Here's the drawing with two shaded views (mm, measured from the low corner). I have some questions. Round coordinates to 2 decimals unless told otherwise and drop trailing zeros. Loops run counter-clockwise (first coordinate to the right, second up) from the corner with the lowest first, then second, coordinate; pieces in that order, holes last.
(1) I want a section at A-A on y = 11.43. Write out the boundary of the cut face in (x, z), plus the area to 3 significant figures.
(2) I want a section at C-C on x = 4. Write out the boundary of the cut face in (y, z), plus the area to 3 significant figures.
(3) If I drill on line 1 along Z through (x, y) = (3.25, 11.43); line 2 along Y through (x, z) = (2.75, 17); line 3 along Y through (x, z) = (1.25, 10.75), over which ranges is the centre line in solid material (lowest first)?
(4) Thinking about a two-plate mould opening in Z: for the marked faces 1, 2 and 3, which applies, released by +Z, released by -Z, zero draft, split by the parting line, or undercut?
(5) Will these pins go through, and if not, where does the flat tip stop? pin 1 Ø1 at (x, y) = (3.5, 12.5) entering from -Z; pin 2 Ø1 at (x, y) = (3, 16.5) entering from +Z.
(6) I want a section at D-D on z = 20.5. Write out the boundary of the cut face in (x, y), plus the area to 3 significant figures.
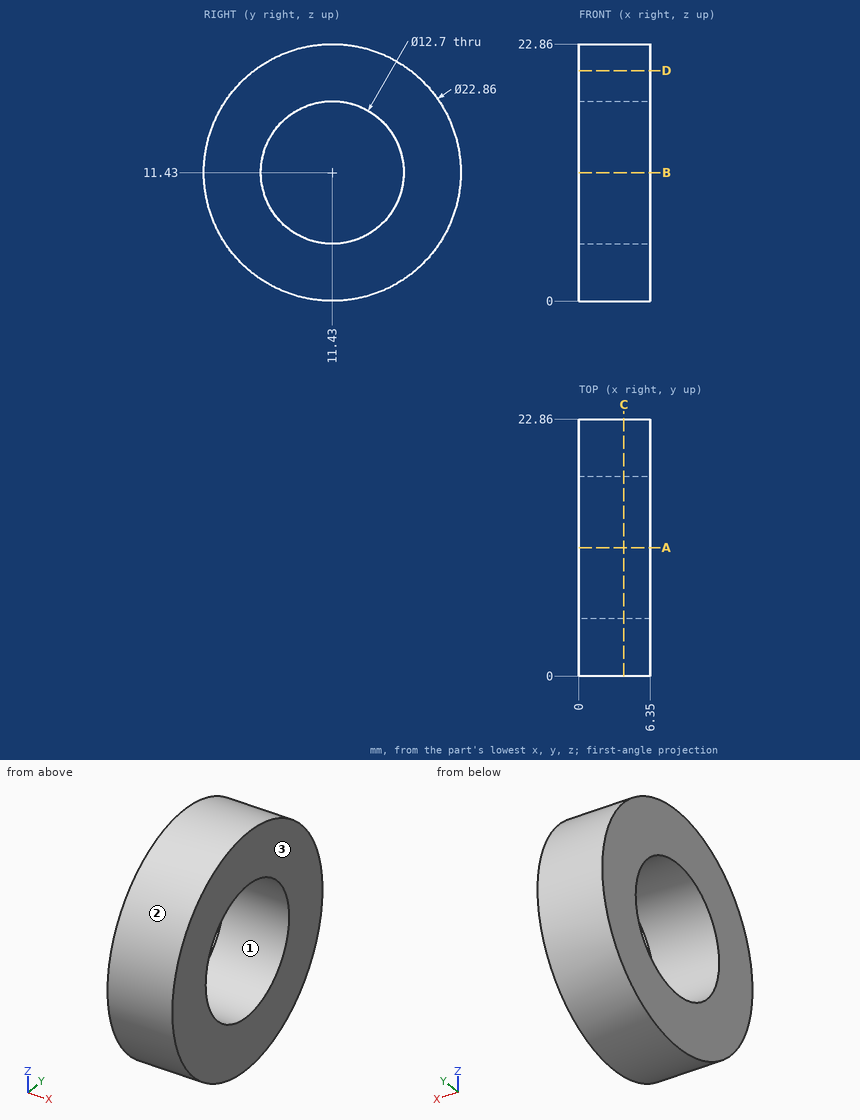
Filled sheet:
1. outline: (0, 0) - (6.35, 0) - (6.35, 5.08) - (0, 5.08) - close; (0, 17.78) - (6.35, 17.78) - (6.35, 22.86) - (0, 22.86) - close
1. area: 64.5 mm2
2. outline: circle Ø22.86 at (11.43, 11.43); hole circle Ø12.7 at (11.43, 11.43)
2. area: 284 mm2
3. line 1: z = 0 to 5.08, 17.78 to 22.86
3. line 2: y = 1.45 to 8.38, 14.48 to 21.41
3. line 3: y = 0.02 to 5.12, 17.74 to 22.84
4. face 1: undercut
4. face 2: split by the parting line
4. face 3: zero draft
5. pin 1: stops at z = 0.01
5. pin 2: stops at z = 21.91
6. outline: (0, 4.47) - (6.35, 4.47) - (6.35, 18.39) - (0, 18.39) - close
6. area: 88.3 mm2
